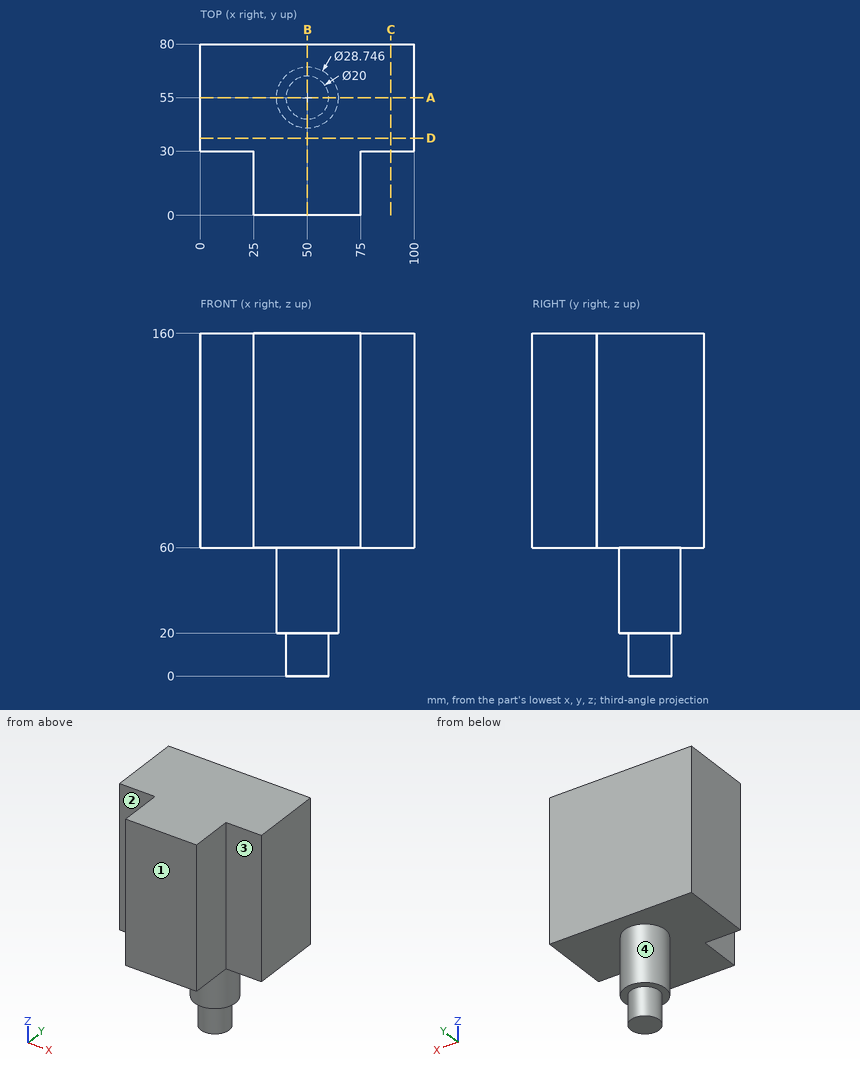
For this review, use the dimensioned drawing (mm, ordinates from the lowest corner) and the shaded views. A direction names the side the tool comes from. Give positions to 0.01 mm unless a question says otherwise; leave off trailing zeros. Order: outer loops, then holes, each group sorted by start corner. A loop starts at its lowest first (then second) coordinate and runs counter-clockwise, first axis right, second up.
1. To check wall thickness, follow L1, parallel to Y at x = 88.5, z = 144; L2, parallel to X at y = 3, z = 153; L3, parallel to Z at x = 34.5, y = 18. State the ranges of each line that lie inside material, in increasing order.
Solution:
L1: y = 30 to 80
L2: x = 25 to 75
L3: z = 60 to 160
2. Add section C-C, the plane x = 89. State the section outline as (y, z) points, then the cut area to 3 significant figures.
Solution:
outline: (30, 60) - (80, 60) - (80, 160) - (30, 160) - close
area: 5,000 mm2
3. Add section D-D, the plane y = 36. State the section outline as (x, z) points, then the cut area to 3 significant figures.
Solution:
outline: (0, 60) - (100, 60) - (100, 160) - (0, 160) - close
area: 10,000 mm2
4. Add section A-A, the plane y = 55. State the section outline as (x, z) points, then the cut area to 4 significant figures.
Solution:
outline: (0, 60) - (35.63, 60) - (35.63, 20) - (40, 20) - (40, 0) - (60, 0) - (60, 20) - (64.37, 20) - (64.37, 60) - (100, 60) - (100, 160) - (0, 160) - close
area: 11,550 mm2
5. Tool access review of the marked faces 1, 2, 3 and 4: name each direction out of +Z, -Z, +X, -X, +Y, -Y from which nothing blocks a thin tool from reaching the whole face with its end or side.
Solution:
face 1: +Z, -Z, +X, -X, -Y
face 2: +Z, -Z, -X, -Y
face 3: +Z, -Z, +X, -Y
face 4: -Z
6. For pin 1 Ø24 at (x, y) = (40.5, 27.5) entering from -Z; pin 2 Ø7.5 at (x, z) = (7, 87.5) entering from -Y; pin 3 Ø12 at (y, z) = (72, 32) entering from -X, all flat-tipped, find the tip position at first contact; note any pin that passes through.
Solution:
pin 1: stops at z = 60
pin 2: stops at y = 30
pin 3: stops at x = 40.75
7. Add section B-B, the plane x = 50. State the section outline as (y, z) points, then the cut area to 3 significant figures.
Solution:
outline: (0, 60) - (40.63, 60) - (40.63, 20) - (45, 20) - (45, 0) - (65, 0) - (65, 20) - (69.37, 20) - (69.37, 60) - (80, 60) - (80, 160) - (0, 160) - close
area: 9,550 mm2
